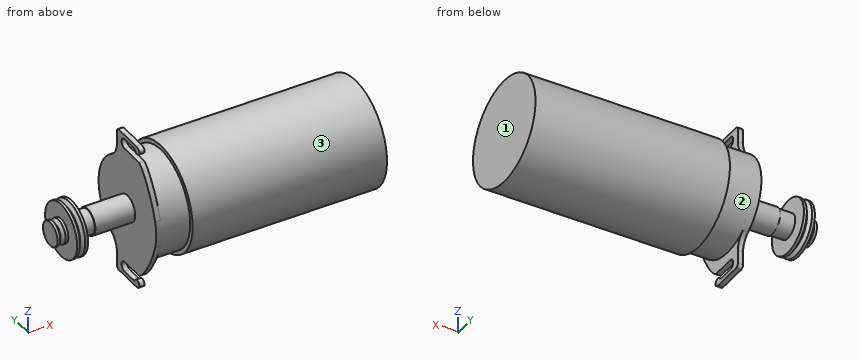
from build123d import *

# Parameters (mm, degrees)
BOSS_EXTRUDE1_DEPTH = 3.9878


with BuildPart() as part:
    # Sketch1 → Revolve3 (revolve)
    with BuildSketch(Plane.XY, mode=Mode.PRIVATE) as revolve3_sk:
        Polygon((65.88246304, 0.116454427), (65.88246304, 40.756454427), (-83.46953696, 40.756454427), (-83.46953696, 37.556054427), (-109.55533696, 37.556054427), (-109.55533696, 10.276454427), (-140.16233696, 10.276454427), (-140.16233696, 9.514454427), (-152.10033696, 9.514454427), (-152.10033696, 20.944454427), (-154.25933696, 20.944454427), (-156.29133696, 17.896454427), (-158.32333696, 20.944454427), (-160.48233696, 20.944454427), (-160.48233696, 9.514454427), (-162.64133696, 9.514454427), (-164.67333696, 6.466454427), (-166.70533696, 9.514454427), (-168.86433696, 9.514454427), (-168.86433696, 0.116454427), align=None)
    revolve(revolve3_sk.sketch.rotate(Axis((-168.86433696, 0.116454427, 0), (1, 0, 0)), 180), axis=Axis((-168.86433696, 0.116454427, 0), (1, 0, 0)))

    # Sketch3 → Boss-Extrude1 (add)
    with BuildSketch(Plane.ZY.offset(109.55533696)):
        with BuildLine():
            Line((43.68878247, 13.702640012), (53.975, 13.702640012))
            ThreePointArc((53.975, 13.702640012), (55.771051224, 12.958691236), (56.515, 11.162640012))
            Line((56.515, 11.162640012), (56.515, -11.153855692))
            add(Edge.make_bspline(
                [(56.515, -11.153855692), (55.734670507, -18.980740225), (46.838290405, -11.919148259), (53.258412532, -9.584126469), (53.213, -7.836402131)],
                knots=[0, 0, 0, 0, 0.643468678, 1, 1, 1, 1], degree=3))
            Line((53.213, -7.836402131), (53.213, 3.905256993))
            ThreePointArc((53.213, 3.905256993), (49.403, 7.715256993), (45.593, 3.905256993))
            Line((45.593, 3.905256993), (45.593, -14.276208246))
            ThreePointArc((45.593, -14.276208246), (45.497523844, -14.966065604), (45.21827309, -15.604060815))
            add(Edge.make_bspline(
                [(45.21827309, -15.604060815), (43.450296459, -18.48702562), (32.758547283, -26.592162263), (21.785194585, -32.669841259), (10.075949561, -35.941816311)],
                knots=[0.01574085, 0.01574085, 0.01574085, 0.01574085, 0.236596649, 1, 1, 1, 1], degree=3))
            ThreePointArc((10.075949561, -35.941816311), (0, -37.323145573), (-10.075949561, -35.941816311))
            add(Edge.make_bspline(
                [(-45.21827309, -15.604060815), (-43.450296459, -18.48702562), (-32.758547283, -26.592162263), (-21.785194585, -32.669841259), (-10.075949561, -35.941816311)],
                knots=[0.01574085, 0.01574085, 0.01574085, 0.01574085, 0.236596649, 1, 1, 1, 1], degree=3))
            ThreePointArc((-45.21827309, -15.604060815), (-45.497523844, -14.966065604), (-45.593, -14.276208246))
            Line((-45.593, -14.276208246), (-45.593, 3.905256993))
            ThreePointArc((-45.593, 3.905256993), (-49.403, 7.715256993), (-53.213, 3.905256993))
            Line((-53.213, 3.905256993), (-53.213, -7.836402131))
            add(Edge.make_bspline(
                [(-56.515, -11.153855692), (-55.734670507, -18.980740225), (-46.838290405, -11.919148259), (-53.258412532, -9.584126469), (-53.213, -7.836402131)],
                knots=[0, 0, 0, 0, 0.643468678, 1, 1, 1, 1], degree=3))
            Line((-56.515, -11.153855692), (-56.515, 11.162640012))
            ThreePointArc((-56.515, 11.162640012), (-55.771051224, 12.958691236), (-53.975, 13.702640012))
            Line((-53.975, 13.702640012), (-43.68878247, 13.702640012))
            ThreePointArc((-43.68878247, 13.702640012), (-36.742018611, 15.475534924), (-31.494435631, 20.360568941))
            ThreePointArc((-31.494435631, 20.360568941), (0, 37.556054427), (31.494435631, 20.360568941))
            ThreePointArc((31.494435631, 20.360568941), (36.742018611, 15.475534924), (43.68878247, 13.702640012))
        make_face()
    extrude(amount=-BOSS_EXTRUDE1_DEPTH)


solid = part.part
The listing builds one solid part. Answer for the finished solid, in the listing's coordinates (mm). Face numbers are marked on the shaded views. Give positions to 0.01 mm unless a question says otherwise; leave off trailing zeros. Write each loop counter-clockwise with the first axis right and the second up, starting at its lowest first coordinate (ties: lowest second). Pieces come first, ordered by that corner, then holes.
1) Find the intervals of material crossed by L1, parallel to X at y = 18, z = 9; L2, parallel to X at y = 2, z = 40; L3, parallel to X at y = 14, z = -13.5, in increasing order.
2) For a pull along X with two mould halves and no side action, classify the marked faces 1, 2 and 3 as pulls with the +X half, pulls with the -X half, needs draft (parallel to the pull), parting line crosses it, or undercut.
3) Section B-B (y = 28) is taken. Write down the section's boundary in (x, z), and give its area (3 significant figures).
4) Given P1, Ø2, axis at x = -108.5, z = 47.5, coming from the +Y side; P2, Ø1, axis at x = -77.5, y = 1.5, coming from the -Z side; P3, Ø24.5, axis at y = -19, z = -19, coming from the -X side, each flat-ended and moving along its own axis, determine where each tip first touches the part or whether it passes through.
5) Section A-A (x = -95) is taken. Write down the section's boundary in (y, z).
6) Section C-C (x = 25) is taken. Write down the section's boundary in (y, z), and give its area (3 significant figures).
Response:
1. L1: x = -160.48 to -157.79, -154.8 to -152.1, -109.56 to 65.88
1. L2: x = -109.56 to -105.57, -83.47 to 65.88
1. L3: x = -160.48 to -157.35, -155.23 to -152.1, -109.56 to 65.88
2. face 1: pulls with the +X half
2. face 2: undercut
2. face 3: needs draft
3. outline: (-109.56, -24.98) - (-83.47, -24.98) - (-83.47, -29.57) - (65.88, -29.57) - (65.88, 29.57) - (-83.47, 29.57) - (-83.47, 24.98) - (-109.56, 24.98) - close
3. area: 10,100 mm2
4. P1: stops at y = 13.7
4. P2: stops at z = -40.63
4. P3: stops at x = -160.48
5. outline: circle Ø74.88 at (0.12, 0)
6. outline: circle Ø81.28 at (0.12, 0)
6. area: 5,190 mm2
